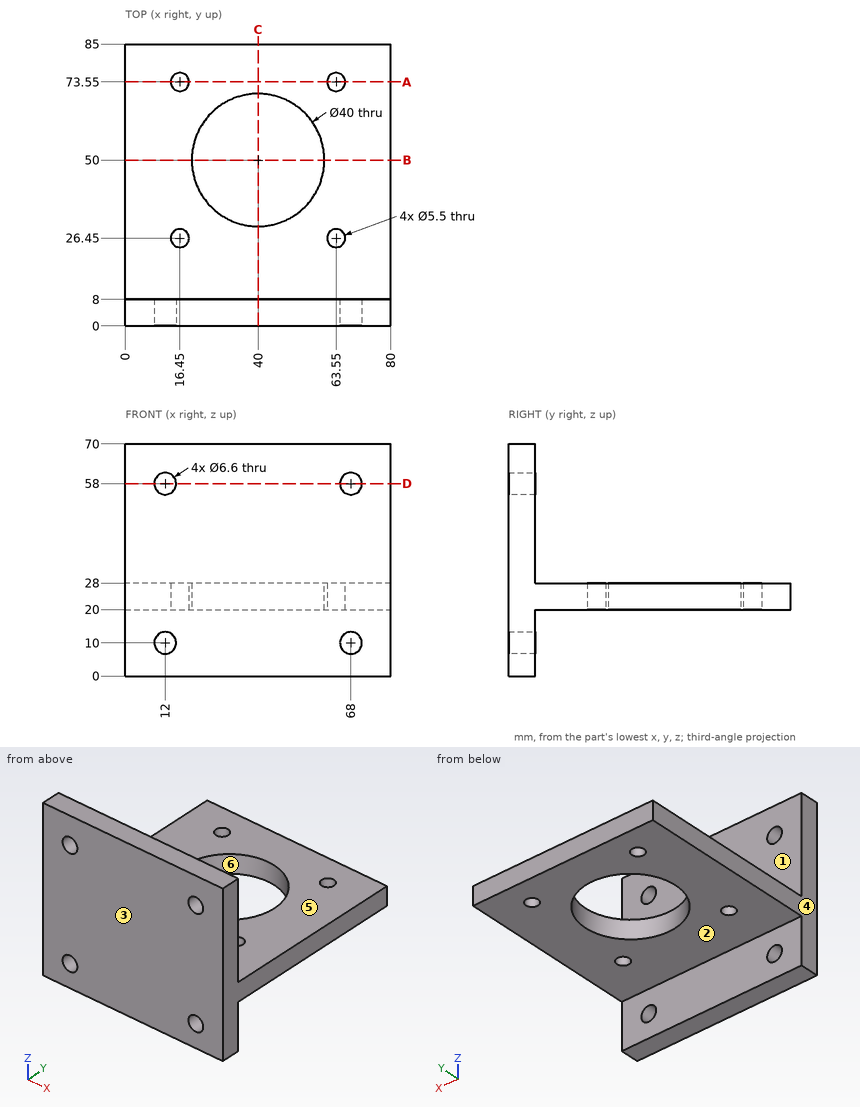
For this review, use the dimensioned drawing (mm, ordinates from the lowest corner) and the shaded views. A direction names the side the tool comes from. Round coordinates to 2 decimals unless told otherwise and drop trailing zeros. Write each loop counter-clockwise with the first axis right and the second up, starting at its lowest first coordinate (ties: lowest second). Pieces come first, ordered by that corner, then holes. Notation, with made-up numbers: M 32.25,0 L 54.25,0 A29 ccw 54.25,29 Z; hole C -17,37.5 d4. An arc over 180 degrees is marked long. Use CSV: the item, a comma, the result in double quotes. Start each with the question number.
(1) For line 1 along Z through (x, y) = (68, 4.75); line 2 along X through (y, z) = (5.5, 58); line 3 along Y through (x, z) = (16.45, 23.25), list the stretches that pass through material, from the lowest coordinate up.
(2) The part is to be moulded in two halves that separate along X. For the marked faces 4, 5 and 6, say which applies: +X half, -X half, draft (parallel to the pull), parting line (faces both ways), or undercut.
(3) We need section B-B, the plane y = 50. State the section outline as (x, z) points.
(4) Clearance check with flat-ended pins moving along their axes: P1, Ø3.5, axis at x = 63.55, y = 26.45, coming from the -Z side; P2, Ø2, axis at x = 62.5, y = 49.5, coming from the +Z side; P3, Ø5, axis at x = 56, z = 52, coming from the +Y side; P4, Ø6.5, axis at x = 63.55, y = 73.55, coming from the -Z side. State where each tip first meets the part, or that it passes through.
(5) We need section D-D, the plane z = 58. State the section outline as (x, y) points.
(6) We need section A-A, the plane y = 73.55. State the section outline as (x, z) points.
(7) Tool access review of the marked faces 1, 2 and 3: name each direction out of +Z, -Z, +X, -X, +Y, -Y from which nothing blocks a thin tool from reaching the whole face with its end or side.
(8) We need section C-C, the plane x = 40. State the section outline as (y, z) points, then the cut area to 3 significant figures.
Findings:
1,line 1,"0 to 6.7, 13.3 to 54.7, 61.3 to 70"
1,line 2,"0 to 8.7, 15.3 to 64.7, 71.3 to 80"
1,line 3,"0 to 23.7, 29.2 to 70.8, 76.3 to 85"
2,face 4,"-X half"
2,face 5,"draft"
2,face 6,"undercut"
3,outline,"M 0,20 L 20,20 L 20,28 L 0,28 Z; M 60,20 L 80,20 L 80,28 L 60,28 Z"
4,P1,"through"
4,P2,"z = 28"
4,P3,"y = 8"
4,P4,"z = 20"
5,outline,"M 0,0 L 8.7,0 L 8.7,8 L 0,8 Z; M 15.3,0 L 64.7,0 L 64.7,8 L 15.3,8 Z; M 71.3,0 L 80,0 L 80,8 L 71.3,8 Z"
6,outline,"M 0,20 L 13.7,20 L 13.7,28 L 0,28 Z; M 19.2,20 L 60.8,20 L 60.8,28 L 19.2,28 Z; M 66.3,20 L 80,20 L 80,28 L 66.3,28 Z"
7,face 1,"+Z, +X, -X, +Y"
7,face 2,"-Z, +X, -X, +Y"
7,face 3,"+Z, -Z, +X, -X, -Y"
8,outline,"M 0,0 L 8,0 L 8,20 L 30,20 L 30,28 L 8,28 L 8,70 L 0,70 Z; M 70,20 L 85,20 L 85,28 L 70,28 Z"
8,area,"856 mm^2"
